Job drawing, mm, ordinate dimensions from the low corner. One solid piece. A direction names the side the tool comes from. Coordinates: 2 decimals unless noted, no trailing zeros. Order: outer loops, then holes, each group sorted by start corner. A loop starts at its lowest first (then second) coordinate and runs counter-clockwise, first axis right, second up. Notation, with made-up numbers: M 19.5,74.25 L 41.5,74.25 A15 cw 41.5,83.25 Z; hole C 44,-28 d4. An arc over 180 degrees is marked long. Write item = value, one per line.
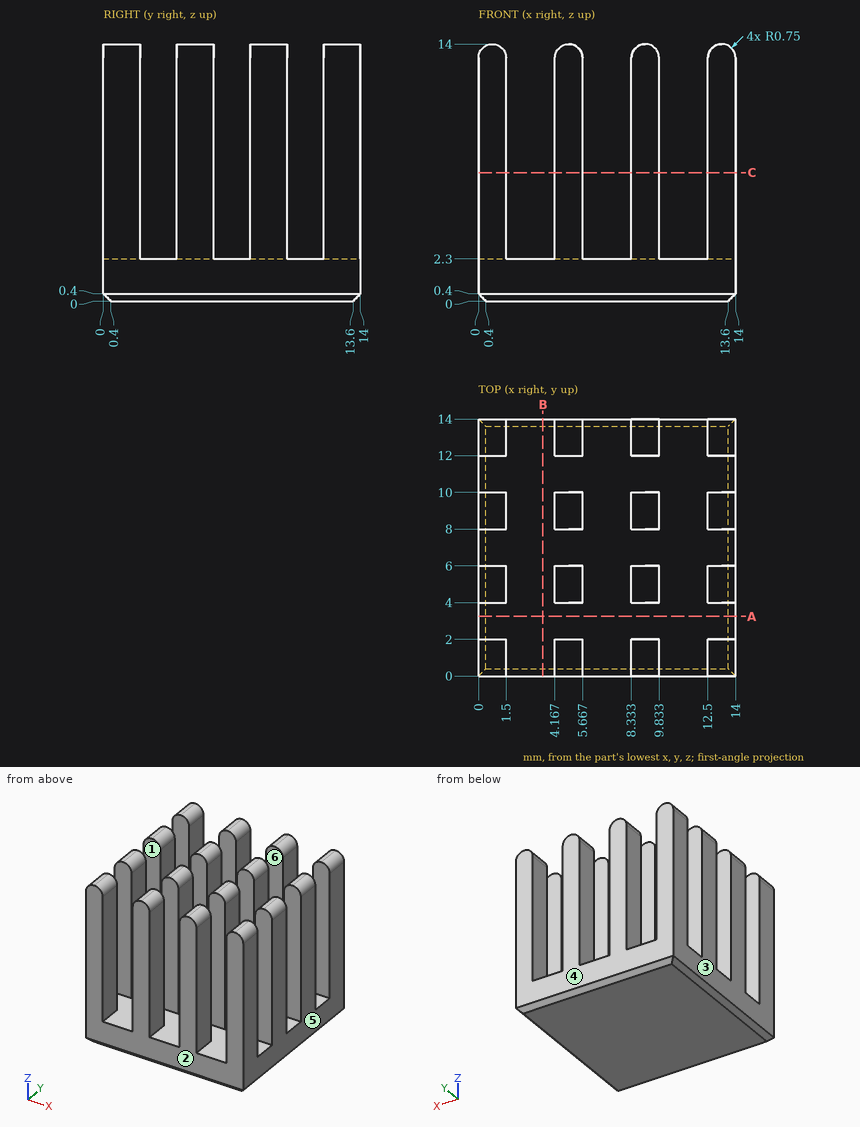
(1) Pull direction Y, two halves, no side cores. Call the marked faces 1, 2, 3 and 4: +Y half, -Y half, draft (parallel to the pull), parting line (faces both ways), or undercut.
Evaluation:
face_1 = undercut
face_2 = -Y half
face_3 = draft
face_4 = +Y half
(2) Tool access for the marked faces 5 and 6: list every direction of +Z, -Z, +X, -X, +Y, -Y with a clear straight run to the whole face (end or side of a thin tool).
Evaluation:
face_5 = +Z, -Z, +X, +Y, -Y
face_6 = +Z, +X, -X
(3) Slice it at A-A, the plane y = 3.25. Write the cut outline in (x, z).
Evaluation:
outline = M 0,0.4 L 0.4,0 L 13.6,0 L 14,0.4 L 14,2.3 L 0,2.3 Z
(4) Slice it at C-C, the plane z = 7. State how many separate pieces and enclosed holes the cut face has.
Evaluation:
separate_pieces = 16
enclosed_holes = 0
(5) Pin check, flat tips, straight feed: pin 1 Ø1.5 at (x, y) = (8, 5.5) entering from +Z; pin 2 Ø2 at (x, y) = (11.5, 7.5) entering from +Z. Stop position of each tip, or through.
Evaluation:
pin_1 = 13.92
pin_2 = 2.3
(6) Wall check: line 1 (X direction, y = 5.25, z = 4); line 2 (Y direction, x = 5.5, z = 9.5); line 3 (Z direction, x = 2.75, y = 5.25). Give the ranges that are in metal, low to high. Write a range as from..to.
Evaluation:
line_1 = 0..1.5, 4.17..5.67, 8.33..9.83, 12.5..14
line_2 = 0..2, 4..6, 8..10, 12..14
line_3 = 0..2.3
